Autodesk Inventor part; units mm, degrees
ref_plane "CP_XY" through (0, 0, 0) normal (1, 0, 0) x (0, 0, -1)
ref_plane "CP_YZ" through (0, 0, 0) normal (0, 0, -1) x (0, 1, 0)
ref_plane "CP_ZX" through (0, 0, 0) normal (0, 1, 0) x (1, 0, 0)
sketch "Sketch_1" plane through (0, 0, 0) normal (0, 0, 1) x (1, 0, 0)
  line L0 (0, 0) -> (-9, 0)
  line L1 (-9, 0) -> (-9, 2.0095)
  line L2 (-9, 2.0095) -> (-8.5095, 2.5)
  line L3 (-8.5095, 2.5) -> (-0.75, 2.5)
  line L4 (-0.75, 2.5) -> (0, 1.75)
  line L5 (0, 1.75) -> (0, 0)
  line L6 (0, 0) -> (-9, 0)
revolve "Revolution1" add sketch "Sketch_1" angle 360 about axis through (0, 0, 0) along (1, 0, 0)
thread "Thread1"
sketch "Sketch_2" plane through (-9, 0, 0) normal (-1, 0, 0) x (0, 1, 0)
  line L0 (-1.25, 0.7217) -> (-1.25, -0.7217)
  line L1 (-1.25, -0.7217) -> (0, -1.4434)
  line L2 (0, -1.4434) -> (1.25, -0.7217)
  line L3 (1.25, -0.7217) -> (1.25, 0.7217)
  line L4 (1.25, 0.7217) -> (0, 1.4434)
  line L5 (0, 1.4434) -> (-1.25, 0.7217)
extrude "Extrusion1" cut sketch "Sketch_2" against normal blind 2
sketch "Sketch_3" plane through (0, 0, 0) normal (0, 0, 1) x (1, 0, 0)
  line L0 (-6.2783, 0) -> (-7, 0)
  line L1 (-7, 0) -> (-7, 1.25)
  line L2 (-7, 1.25) -> (-6.2783, 0)
  line L3 (-6.2783, 0) -> (-7, 0)
revolve "Revolution2" cut sketch "Sketch_3" angle 360 about axis through (-6.2783, 0, 0) along (1, 0, 0)
ref_plane "CP_XY" through (0, 0, 0) normal (1, 0, 0) x (0, 0, -1)
ref_plane "CP_YZ" through (0, 0, 0) normal (0, 0, -1) x (0, 1, 0)
ref_plane "CP_ZX" through (0, 0, 0) normal (0, 1, 0) x (1, 0, 0)
properties part number "SET-SCREW5-9"
Work out the finished part from the listing and answer in its coordinate system (mm). Give positions to 0.01 mm unless a question says otherwise; leave off trailing zeros. Write each loop counter-clockwise with the first axis right and the second up, starting at its lowest first coordinate (ties: lowest second). Pieces come first, ordered by that corner, then holes. Notation, with made-up numbers: (-28.75, -34) - (11.25, -34) arc R23 cw to (11.25, -23) - close; hole circle Ø5 at (16, 65.5). An arc over 180 degrees is marked (long way). One line per item, written item: value. Start each with the question number.
1. Find section A-A (x = -8). Write down the section's boundary in (y, z).
2. Find section B-B (x = -1.25). Write down the section's boundary in (y, z).
3. Given pin 1 (0.7 mm diameter, centred on y = 0, z = -1, fed in from -X), flat-ended and moving along its own axis, determine where the tip first touches the part or whether it passes through.
4. Consider probe 1 along Z at (x, y) = (-8, -0.8); probe 2 along X at (y, z) = (0.75, 1.95); probe 3 along Y at (x, z) = (-6, 0.7). Determine where each line is inside the solid, lowest interval first.
5. For a pull along Z with two mould halves and no side action, classify faces 1 (the cylindrical face through (-4.58, -0.54, -2.44)), 2 (the flat face through (0, 0, 0)), 3 (the flat face through (-8.01, -0.63, 1.08)) as +Z half, -Z half, draft (parallel to the pull), parting line (faces both ways), or undercut.
6. Find section C-C (x = -0.25). Write down the section's boundary in (y, z).
Geometry results:
1. outline: circle Ø5 at (0, 0); hole (-1.25, -0.72) - (0, -1.44) - (1.25, -0.72) - (1.25, 0.72) - (0, 1.44) - (-1.25, 0.72) - close
2. outline: circle Ø5 at (0, 0)
3. pin 1: x = -7
4. probe 1: -2.37 to -0.98, 0.98 to 2.37
4. probe 2: -8.92 to -0.34
4. probe 3: -2.4 to 2.4
5. face 1: parting line
5. face 2: draft
5. face 3: undercut
6. outline: circle Ø4 at (0, 0)
